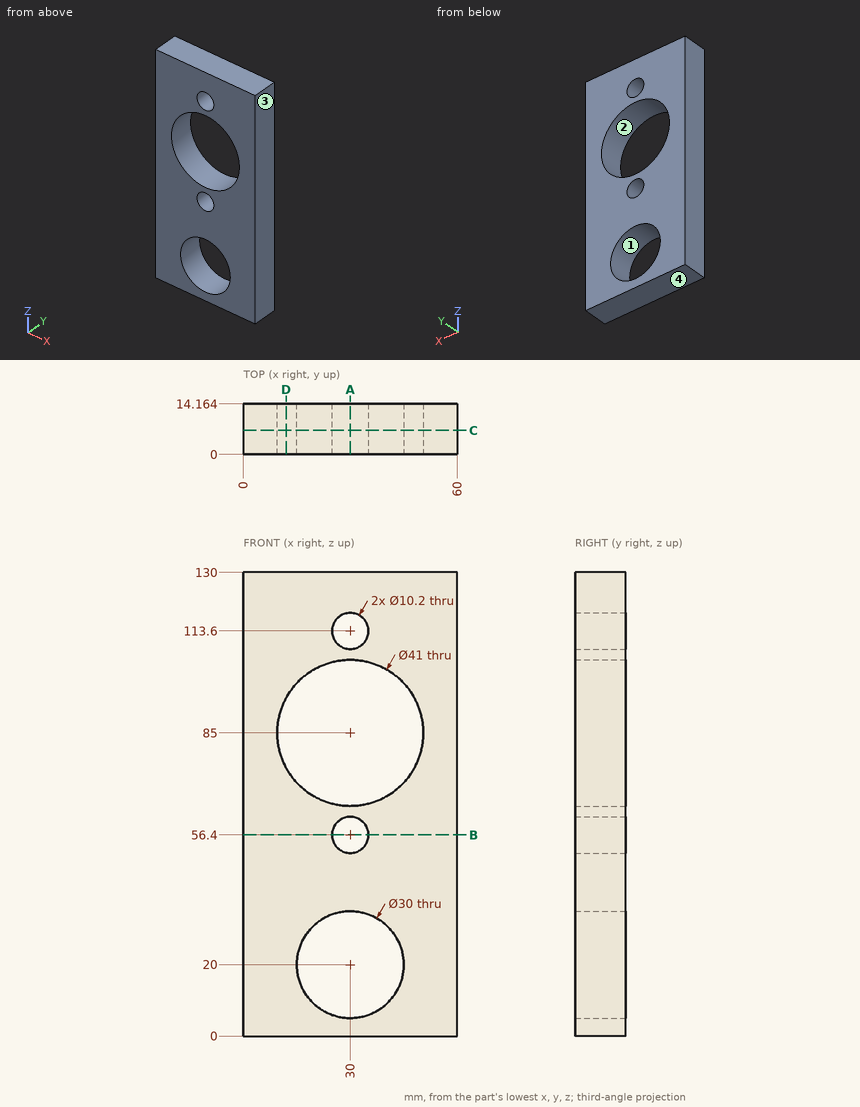
Verification items for this drawing (mm, ordinates from the low corner). Give positions to 0.01 mm unless a question says otherwise; leave off trailing zeros. Write each loop counter-clockwise with the first axis right and the second up, starting at its lowest first coordinate (ties: lowest second). Pieces come first, ordered by that corner, then holes. Notation, with made-up numbers: (62, 64.5) -> (108, 64.5) arc R14 cw to (108, 72.5) -> close; hole circle Ø8 at (4.25, 55). An arc over 180 degrees is marked (long way). Use CSV: the item, a comma, the result in double quotes. Start each with the question number.
Q1. Cross-section at C-C on y = 6.75. Enter the section's corners in (x, z).
Q2. Cross-section at A-A on x = 30. Enter the section's corners in (y, z).
Q3. Scan lines: line 1 along Z through (x, y) = (30, 6.25); line 2 along X through (y, z) = (8.25, 113.6); line 3 along X through (y, z) = (9.25, 20). Record each from-to range of solid material in increasing order.
Q4. Release check for a two-part mould opening along Z. For the marked faces 1, 2, 3 and 4 record: +Z half, -Z half, draft (parallel to the pull), parting line (faces both ways), or undercut.
Q5. Cross-section at D-D on x = 12. Enter the section's corners in (y, z), and give its area (3 significant figures).
Q6. Cross-section at B-B on z = 56.4. Enter the section's corners in (x, y).
Working result:
1,outline,"(0, 0) -> (60, 0) -> (60, 130) -> (0, 130) -> close; hole circle Ø41 at (30, 85); hole circle Ø30 at (30, 20); hole circle Ø10.2 at (30, 56.4); hole circle Ø10.2 at (30, 113.6)"
2,outline,"(0, 0) -> (14.16, 0) -> (14.16, 5) -> (0, 5) -> close; (0, 35) -> (14.16, 35) -> (14.16, 51.3) -> (0, 51.3) -> close; (0, 61.5) -> (14.16, 61.5) -> (14.16, 64.5) -> (0, 64.5) -> close; (0, 105.5) -> (14.16, 105.5) -> (14.16, 108.5) -> (0, 108.5) -> close; (0, 118.7) -> (14.16, 118.7) -> (14.16, 130) -> (0, 130) -> close"
3,line 1,"z = 0 to 5, 35 to 51.3, 61.5 to 64.5, 105.5 to 108.5, 118.7 to 130"
3,line 2,"x = 0 to 24.9, 35.1 to 60"
3,line 3,"x = 0 to 15, 45 to 60"
4,face 1,"undercut"
4,face 2,"undercut"
4,face 3,"draft"
4,face 4,"-Z half"
5,outline,"(0, 0) -> (14.16, 0) -> (14.16, 75.19) -> (0, 75.19) -> close; (0, 94.81) -> (14.16, 94.81) -> (14.16, 130) -> (0, 130) -> close"
5,area,"1,560 mm^2"
6,outline,"(0, 0) -> (24.9, 0) -> (24.9, 14.16) -> (0, 14.16) -> close; (35.1, 0) -> (60, 0) -> (60, 14.16) -> (35.1, 14.16) -> close"
